from build123d import *

# Parameters (mm, degrees)
F0_R           = 20
F1_DEPTH       = 2
F2_R           = 5
F3_DEPTH       = 30
F6_DEPTH       = 12
F7_R           = 2.25
F8_DEPTH       = 1.5
F8_DEPTH_BACK  = 6.5
F10_DEPTH      = 17.501
F10_DEPTH_BACK = 22.501
F12_DEPTH      = 2.2
F12_DEPTH_BACK = 2.2
F15_R          = 3
F16_DEPTH      = 15


# Not quite as in the source:
# - a pattern or mirror of a feature is missing from the dataset's text; its kind, count and spacing are read off the source's solid


with BuildPart() as f1:
    # F0 (on Front) → F1 (new body)
    with BuildSketch(Plane.XZ):
        Circle(F0_R)
    extrude(amount=F1_DEPTH)

    # F2 (on face) → F3 (join)
    with BuildSketch(Plane.XZ.offset(2)):
        Circle(F2_R)
    extrude(amount=F3_DEPTH)

    # F5 (on face) → F6 (cut)
    with BuildSketch(Plane.XZ.offset(32)):
        with BuildLine():
            Line((4.3301270189, 2.5), (-4.3301270189, 2.5))
            ThreePointArc((-4.3301270189, 2.5), (-4.8296291314, 1.2940952255), (-5, 0))
            ThreePointArc((-5, 0), (-4.8296291314, -1.2940952255), (-4.3301270189, -2.5))
            Line((-4.3301270189, -2.5), (4.3301270189, -2.5))
            ThreePointArc((4.3301270189, -2.5), (4.8296291314, -1.2940952255), (5, 0))
            ThreePointArc((5, 0), (4.8296291314, 1.2940952255), (4.3301270189, 2.5))
        make_face()
    extrude(amount=-F6_DEPTH, mode=Mode.SUBTRACT)

    # F7 (on face) → F8 (cut, two sides)
    with BuildSketch(Plane(origin=(0, 0, 2.5), x_dir=(1, 0, 0), z_dir=(0, 0, -1))) as f8_sk:
        with Locations((0, 27)):
            Circle(F7_R)
    extrude(amount=-F8_DEPTH, mode=Mode.SUBTRACT)
    extrude(f8_sk.sketch, amount=F8_DEPTH_BACK, mode=Mode.SUBTRACT)

    # F9 (on face) → F10 (cut, two sides)
    with BuildSketch(Plane.XY.offset(-2.5)) as f10_sk:
        with BuildLine():
            Line((4.3301270189, -32), (4.3301270189, -29.5))
            ThreePointArc((4.3301270189, -29.5), (2.5, -31.3301270189), (0, -32))
            Line((0, -32), (4.3301270189, -32))
        make_face()
        with BuildLine():
            Line((-4.3301270189, -32), (0, -32))
            ThreePointArc((0, -32), (-2.5, -31.3301270189), (-4.3301270189, -29.5))
            Line((-4.3301270189, -29.5), (-4.3301270189, -32))
        make_face()
    extrude(amount=-F10_DEPTH, mode=Mode.SUBTRACT)
    extrude(f10_sk.sketch, amount=F10_DEPTH_BACK, mode=Mode.SUBTRACT)

    # F11 (on Right) → F12 (cut, two sides)
    with BuildSketch(Plane.YZ) as f12_sk:
        Polygon((-32, 2.5), (-29.5, 2.5), (-29.4072434941, 3.0565390355), (-32, 3.8), align=None)
        Polygon((-29.5, 2.5), (-27.466361223, 2.5), (-29.4072434941, 3.0565390355), align=None)
    f12 = extrude(amount=-F12_DEPTH, mode=Mode.SUBTRACT) + extrude(f12_sk.sketch, amount=F12_DEPTH_BACK, mode=Mode.SUBTRACT)

    # F12_copies: F12 across plane
    add(f12.mirror(Plane(origin=(0, 0, 0), x_dir=(-1, 0, 0), z_dir=(0, 0, -1))), mode=Mode.SUBTRACT)

    # F15 (on offset) → F16 (cut, through all)
    with BuildSketch(Plane.XZ.offset(17)):
        Circle(F15_R)
    extrude(amount=-F16_DEPTH, mode=Mode.SUBTRACT)


solid = f1.part
Source: CAD feature listing. Evaluate the final solid. Frame: model axes, mm. A direction names the side the tool comes from. Give positions to 0.01 mm unless a question says otherwise; leave off trailing zeros. Loops run counter-clockwise (first coordinate to the right, second up) from the corner with the lowest first, then second, coordinate; pieces in that order, holes last. Notation, with made-up numbers: (83, 2.5) -> (121, 2.5) arc R20 cw to (121, 12.5) -> close; hole circle Ø6 at (48.5, -12). An arc over 180 degrees is marked (long way). Use a Markdown table: item, result. Add a question column.
1) First-contact query: pin 1 (3.5 mm diameter, centred on x = -1, y = -26.5, fed in from +Z); pin 2 (6 mm diameter, centred on y = -24.5, z = -2.5, fed in from -X); pin 3 (1.3 mm diameter, centred on y = -30.5, z = 3, fed in from -X); pin 4 (1.5 mm diameter, centred on x = -6, y = -3.5, fed in from -Z). Flat tips, straight axial feed; report the tip coordinate or a pass-through.
2) Line query: line 1 along Z through (x, y) = (0, -14); line 2 along X through (y, z) = (-27, 3.25); line 3 along Z through (x, y) = (-2.5, -30). Output: solid intervals per line, ascending. Write a range as [from, to].
3) Reachability of faces 4 (the face through (0, -17, 0)), 5 (the face through (2.2, -30, -3)), 6 (the face through (0.1, -24.5, 2.5)), 7 (the face through (-4.336, -0.986, -19.524)) from +Z, -Z, +X, -X, +Y, -Y: full face, straight path, thin tool, end or side. Return the list, or none.
4) Section query C-C, the plane z = -12. Return the cut outline in (x, y), then the cut area to 3 significant figures.
5) Section query A-A, the plane y = -26. Return the cut outline in (x, z), then the cut area to 3 significant figures.
6) Pull-direction query (Y, two-part tool) for faces 1 (the face through (-0.1, -24.5, -2.5)), 2 (the face through (0, -2, 0)), 3 (the face through (0, -20, 0)); classes: +Y half, -Y half, draft (parallel to the pull), parting line (faces both ways), or undercut.
7) Section query B-B, the plane z = 0. Return the cut outline in (x, y).
8) Section query D-D, the plane y = -16. Return the cut outline in (x, z), then the cut area to 3 significant figures.
Numbers:
| question | item | result |
|---|---|---|
| 1 | pin 1 | stops at z = 5 |
| 1 | pin 2 | stops at x = -4.33 |
| 1 | pin 3 | stops at x = -4.1 |
| 1 | pin 4 | passes through |
| 2 | line 1 | z = [-5, -3], [3, 5] |
| 2 | line 2 | x = [-3.8, -2.25], [2.25, 3.8] |
| 2 | line 3 | z = [-4.33, -2.5], [2.5, 4.33] |
| 3 | face 4 | none |
| 3 | face 5 | -Y |
| 3 | face 6 | +X, -X, -Y |
| 3 | face 7 | +Y, -Y |
| 4 | outline | (-16, -2) -> (16, -2) -> (16, 0) -> (-16, 0) -> close |
| 4 | area | 64.0 mm2 |
| 5 | outline | (-4.33, -2.5) arc R5 ccw to (4.33, -2.5) -> (2.02, -2.5) -> (2.02, -4) -> (-2.02, -4) -> (-2.02, -2.5) -> close; (-4.33, 2.5) -> (-2.02, 2.5) -> (-2.02, 4) -> (2.02, 4) -> (2.02, 2.5) -> (4.33, 2.5) arc R5 ccw to start |
| 5 | area | 18.6 mm2 |
| 6 | face 1 | draft |
| 6 | face 2 | undercut |
| 6 | face 3 | -Y half |
| 7 | outline | (-20, -2) -> (-5, -2) -> (-5, -20) -> (5, -20) -> (5, -2) -> (20, -2) -> (20, 0) -> (-20, 0) -> close; hole (-3, -17) -> (3, -17) -> (3, -2) -> (-3, -2) -> close |
| 8 | outline | circle Ø10 at (0, 0); hole circle Ø6 at (0, 0) |
| 8 | area | 50.3 mm2 |
